Can you work these out from the model? Positions are in its coordinate system, mm. Coordinates: 2 decimals unless noted, no trailing zeros. Order: outer loops, then holes, each group sorted by start corner. A loop starts at its lowest first (then second) coordinate and runs counter-clockwise, first axis right, second up. Notation, with made-up numbers: (-21.5, -23.75) - (2.5, -23.75) arc R20 ccw to (2.5, -2.75) - close; hole circle Ø1 at (7.5, -32). An arc over 180 degrees is marked (long way). Return JSON: item names as keys, results as strings. Group by question number.
1) Imagine slicing it at B-B (z = 0). Write out the boundary of the cut face in (x, y) (3 decimals).
2) If we mould it in two halves opening along Z, with no side actions, what happens to faces 1 (the face through (42.33, 0.99, -3.03)), 2 (the face through (-24, 0, 0))? For each: pulls with the +Z half, pulls with the -Z half, needs draft (parallel to the pull), parting line crosses it, or undercut.
3) Imagine slicing it at D-D (x = 45.5). Write out the boundary of the cut face in (y, z), and give its area (3 significant figures).
4) Imagine slicing it at C-C (y = 0.9). Write out the boundary of the cut face in (x, z) (3 decimals), and give its area (3 significant figures).
5) Imagine slicing it at A-A (x = 85). Write out the boundary of the cut face in (y, z).
6) If I drill on line 1 along X through (y, z) = (0.75, 0) (3 decimals); line 2 along X through (y, z) = (0.45, 1.75), over which ranges is the centre line in solid material (lowest first)?
```python
from build123d import *

# Parameters (mm, degrees)
SKETCH1_W           = 200
SKETCH1_H           = 30
SKETCH1_R           = 14
BOSS_EXTRUDE3_DEPTH = 2
SKETCH1_7_R         = 3.185
CUT_EXTRUDE1_DEPTH  = 10


with BuildPart() as part:
    # Sketch1 → Boss-Extrude3 (new body)
    with BuildSketch(Plane(origin=(0, 0, 0), x_dir=(1, 0, 0), z_dir=(0, 1, 0))):
        Rectangle(SKETCH1_W, SKETCH1_H)
        with Locations(Location((85, 0, 0), (0, 0, 270))):
            Circle(SKETCH1_R, mode=Mode.SUBTRACT)
        with Locations(Location((56, 0, 0), (0, 0, 270))):
            Circle(SKETCH1_R, mode=Mode.SUBTRACT)
    extrude(amount=BOSS_EXTRUDE3_DEPTH)

    # Sketch1_7 → Cut-Extrude1 (cut)
    with BuildSketch(Plane(origin=(0, 0, 0), x_dir=(1, 0, 0), z_dir=(0, 1, 0))):
        with Locations((-100, 0)):
            Circle(SKETCH1_7_R)
    extrude(amount=CUT_EXTRUDE1_DEPTH, mode=Mode.SUBTRACT)


solid = part.part
```
Calculated:
{
 "1": {"outline": "(-96.815, 0) - (42, 0) - (42, 2) - (-96.815, 2) - close; (70, 0) - (71, 0) - (71, 2) - (70, 2) - close; (99, 0) - (100, 0) - (100, 2) - (99, 2) - close"},
 "2": {"face 1": "undercut", "face 2": "needs draft"},
 "3": {"outline": "(0, -15) - (2, -15) - (2, -9.26) - (0, -9.26) - close; (0, 9.26) - (2, 9.26) - (2, 15) - (0, 15) - close", "area": "23.0 mm2"},
 "4": {"outline": "(-100, -15) - (100, -15) - (100, 15) - (-100, 15) - (-100, 3.185) arc R3.185 cw to (-100, -3.185) - close; hole circle Ø28 at (56, 0); hole circle Ø28 at (85, 0)", "area": "4,750 mm2"},
 "5": {"outline": "(0, -15) - (2, -15) - (2, -14) - (0, -14) - close; (0, 14) - (2, 14) - (2, 15) - (0, 15) - close"},
 "6": {"line 1": "-96.815 to 42, 70 to 71, 99 to 100", "line 2": "-97.34 to 42.11, 69.89 to 71.11, 98.89 to 100"}
}
